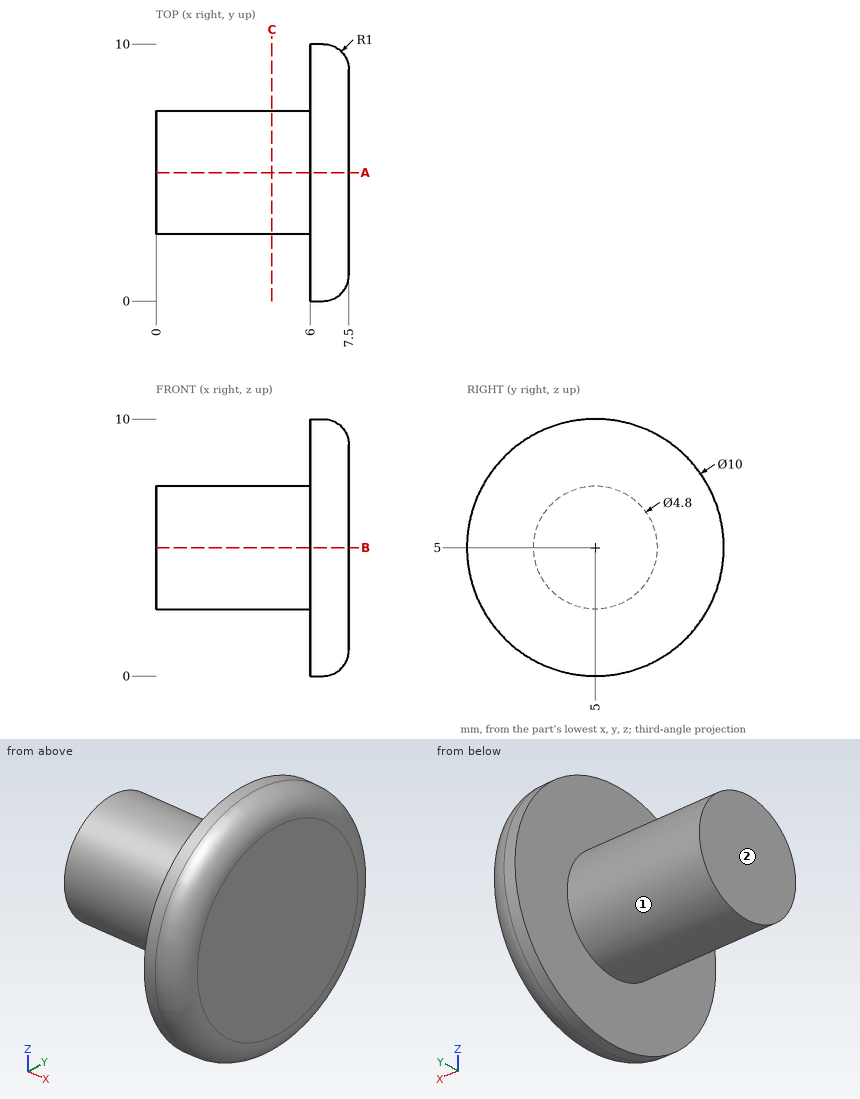
Could you check a few things on this drawing? It's one solid part, dimensions in mm from its lowest x, y, z. A direction names the side the tool comes from. Coordinates: 2 decimals unless noted, no trailing zeros. Order: outer loops, then holes, each group sorted by start corner. A loop starts at its lowest first (then second) coordinate and runs counter-clockwise, first axis right, second up. Notation, with made-up numbers: M 6.25,-14 L 57.25,-14 A34 cw 57.25,19 Z; hole C 1.5,37.5 d1. An arc over 180 degrees is marked long. Use a Markdown table: item, result. Add a question column.
Q1. I want a section at C-C on x = 4.5. List the corners of the cut face in (y, z) for me.
Q2. I want a section at A-A on y = 5. List the corners of the cut face in (x, z) for me, then the cut area to 3 significant figures.
Q3. If I drill on L1, parallel to X at y = 8.5, z = 5.25; L2, parallel to Z at x = 7, y = 5.25; L3, parallel to Y at x = 4, z = 5.5, over which ranges is the centre line in solid material (lowest first)?
Q4. I'm going to push a flat-ended pin straight in: pin 1 (4 mm diameter, centred on x = 2.5, z = 9, fed in from -Y). Where does the tip first touch, or does it pass through?
Q5. Which directions (+Z, -Z, +X, -X, +Y, -Y) give clear straight access to the entire face, cutting with the end or side of a thin tool? Please do the marked faces 1 and 2.
Checked values:
| question | item | result |
|---|---|---|
| 1 | outline | C 5,5 d4.8 |
| 2 | outline | M 0,2.6 L 6,2.6 L 6,0 L 6.5,0 A1 ccw 7.5,1 L 7.5,9 A1 ccw 6.5,10 L 6,10 L 6,7.4 L 0,7.4 Z |
| 2 | area | 43.4 mm² |
| 3 | L1 | 6 to 7.5 |
| 3 | L2 | 0.14 to 9.86 |
| 3 | L3 | 2.65 to 7.35 |
| 4 | pin 1 | y = 3.67 |
| 5 | face 1 | -X |
| 5 | face 2 | +Z, -Z, -X, +Y, -Y |
